Build history of the part. All positions in model axes, mm. Face numbers are marked on the shaded views. Round coordinates to 2 decimals unless told otherwise and drop trailing zeros. Order: outer loops, then holes, each group sorted by start corner. A loop starts at its lowest first (then second) coordinate and runs counter-clockwise, first axis right, second up. Notation, with made-up numbers: (23.25, -34.75) -> (79.25, -34.75) arc R20 ccw to (79.25, 2.25) -> close; hole circle Ø5 at (61, 69.25). An arc over 180 degrees is marked (long way). Answer as a JSON object with one key per item and string values.
from build123d import *

# Parameters (mm, degrees)
F0_R     = 19
F0_R_2   = 12.5
F1_DEPTH = 5.75
F0_R_3   = 11.1
F2_DEPTH = 7.05
F3_SIZE  = 0.6
F4_SIZE  = 0.6


with BuildPart() as f1:
    # F0 (on Top) → F1 (new body)
    with BuildSketch(Plane.XY):
        with Locations((-89.7258073092, 31.1653446406)):
            Circle(F0_R)
        with Locations((-89.7258073092, 31.1653446406)):
            Circle(F0_R_2, mode=Mode.SUBTRACT)
    extrude(amount=F1_DEPTH)

    # F0 (on Top) → F2 (join)
    with BuildSketch(Plane.XY):
        with Locations((-89.7258073092, 31.1653446406)):
            Circle(F0_R_2)
        with Locations((-89.7258073092, 31.1653446406)):
            Circle(F0_R_3, mode=Mode.SUBTRACT)
    extrude(amount=F2_DEPTH)

    # F3
    f3_edges = [f1.edges().sort_by_distance(p)[0] for p in [
        (-108.725807, 31.165345, 5.75),
        (-108.725807, 31.165345, 0),
    ]]
    chamfer(f3_edges, length=F3_SIZE)

    # F4
    f4_edges = [f1.edges().sort_by_distance(p)[0] for p in [
        (-108.725807, 31.165345, 5.15),
        (-108.725807, 31.165345, 0.6),
    ]]
    chamfer(f4_edges, length=F4_SIZE)


solid = f1.part
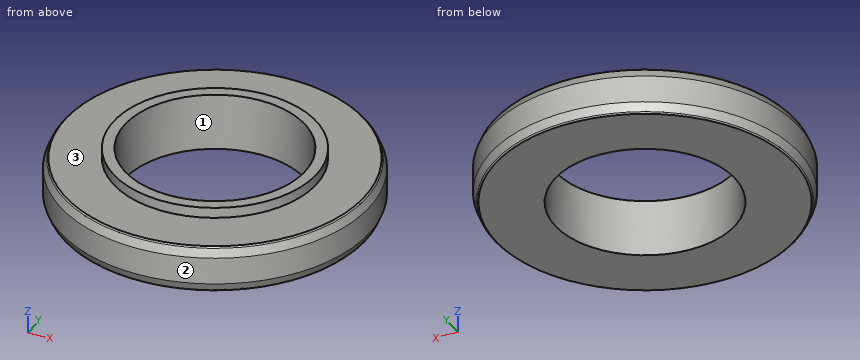
1) Pull direction Y, two halves, no side cores. Call the marked faces 1, 2 and 3: pulls with the +Y half, pulls with the -Y half, needs draft (parallel to the pull), parting line crosses it, or undercut.
Checked values:
{"face 1": "undercut", "face 2": "parting line crosses it", "face 3": "needs draft"}
2) Cut at A-A, the plane z = 3.75. Give the cut face in (x, y), plus the area to 3 significant figures.
Checked values:
{"outline": "circle Ø38 at (-89.73, 31.17); hole circle Ø22.2 at (-89.73, 31.17)", "area": "747 mm²"}
3) Probe L1, parallel to Z at x = -95.5, y = 18; L2, parallel to X at y = 32.5, z = 6; L3, parallel to Y at x = -91.5, z = 5. List the from-to ranges inside material, lowest first. Write a range as from..to.
Checked values:
{"L1": "z = 0..5.75", "L2": "x = -102.15..-100.75, -78.71..-77.3", "L3": "y = 12.44..20.21, 42.12..49.9"}
4) Flat gauge pins, fed straight in: pin 1 Ø1 at (x, z) = (-97.5, 2) entering from +Y; pin 2 Ø8 at (x, y) = (-80.5, 26) entering from +Z; pin 3 Ø20 at (x, y) = (-89.73, 31.17) entering from -Z; pin 4 Ø5 at (x, y) = (-104, 39) entering from +Z. Where does each tip first touch, or does it go through?
Checked values:
{"pin 1": "stops at y = 48.72", "pin 2": "stops at z = 7.05", "pin 3": "passes through", "pin 4": "stops at z = 5.75"}
